Study the drawing (mm; zero at the part's minimum x, y, z) and answer. A direction names the side the tool comes from. Coordinates: 2 decimals unless noted, no trailing zeros. Loops run counter-clockwise (first coordinate to the right, second up) from the corner with the lowest first, then second, coordinate; pieces in that order, holes last.
Q1. Section B-B (z = 9) is taken. Give the vertices of the cut face in (x, y), then the cut area to 3 significant figures.
Q2. The mould has two halves that part along X. Classify the marked faces 1, 2 and 3: pulls with the +X half, pulls with the -X half, needs draft (parallel to the pull), parting line crosses it, or undercut.
Q3. Section A-A (x = 97.5) is taken. Give the vertices of the cut face in (y, z), then the cut area to 3 significant figures.
Q4. Which of the six approach directions +Z, -Z, +X, -X, +Y, -Y give full straight-line access (tool end or side, diameter ignored) to the marked faces 4, 5, 6 and 7?
Q5. Section C-C (x = 12.5) is taken. Give the vertices of the cut face in (y, z), then the cut area to 3 significant figures.
Q6. Flat-ended cylindrical pins translate along their axes: P1, Ø7, axis at x = 97.5, z = 12.5, coming from the +Y side; P2, Ø5, axis at x = 85, z = 16.5, coming from the +Y side; P3, Ø8, axis at x = 20, y = 8, coming from the -Z side; P4, Ø10, axis at x = 92, z = 10, coming from the +Y side. Find the tip coordinate at first contact, or state that the pin passes through.
Q7. Section D-D (y = 1.5) is taken. Give the vertices of the cut face in (x, z) (1 decimal).
Q8. Straight lines are drawn through the part: line 1 (Z direction, x = 12.5, y = 11.25); line 2 (Z direction, x = 97.5, y = 2); line 3 (Z direction, x = 46.5, y = 8.5). For each, find the intervals that lie inside material, in ascending order.
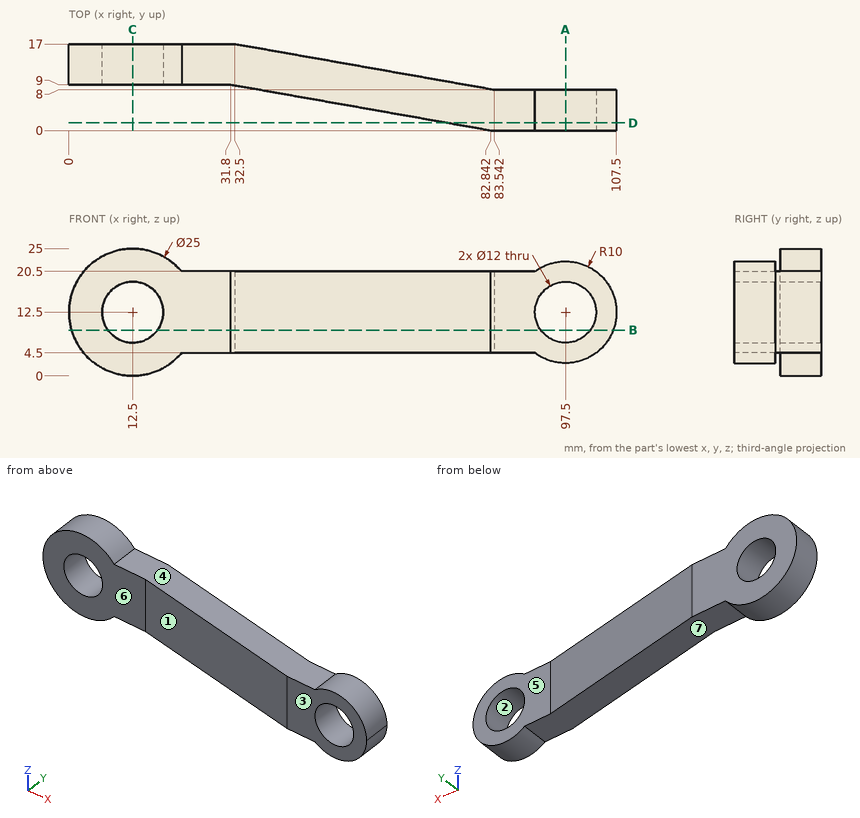
Numbers:
1. outline: (0.5, 9) - (7.63, 9) - (7.63, 17) - (0.5, 17) - close; (17.37, 9) - (31.8, 9) - (82.84, 0) - (92.63, 0) - (92.63, 8) - (83.54, 8) - (32.5, 17) - (17.37, 17) - close; (102.37, 0) - (106.87, 0) - (106.87, 8) - (102.37, 8) - close
1. area: 701 mm2
2. face 1: pulls with the -X half
2. face 2: undercut
2. face 3: needs draft
3. outline: (0, 2.5) - (8, 2.5) - (8, 6.5) - (0, 6.5) - close; (0, 18.5) - (8, 18.5) - (8, 22.5) - (0, 22.5) - close
3. area: 64.0 mm2
4. face 4: +Z, +Y, -Y
4. face 5: +Z, -Z, +X, +Y
4. face 6: +Z, -Z, -X, -Y
4. face 7: -Z, +Y, -Y
5. outline: (9, 0) - (17, 0) - (17, 6.5) - (9, 6.5) - close; (9, 18.5) - (17, 18.5) - (17, 25) - (9, 25) - close
5. area: 104 mm2
6. P1: passes through
6. P2: stops at y = 8.18
6. P3: stops at z = 0.54
6. P4: stops at y = 8
7. outline: (74.3, 4.5) - (91.5, 4.5) arc R10 ccw (long way) to (91.5, 20.5) - (74.3, 20.5) - close; hole circle Ø12 at (97.5, 12.5)
8. line 1: z = 0 to 6.5, 18.5 to 25
8. line 2: z = 2.5 to 6.5, 18.5 to 22.5
8. line 3: z = 4.5 to 20.5
